Build history of the part. All positions in model axes, mm. A direction names the side the tool comes from. Give positions to 0.01 mm unless a question says otherwise; leave off trailing zeros. Order: outer loops, then holes, each group sorted by start corner. A loop starts at its lowest first (then second) coordinate and runs counter-clockwise, first axis right, second up. Notation, with made-up numbers: (-14, 79.5) - (19, 79.5) arc R31 cw to (19, 117.5) - close; hole circle Ø2 at (48.5, 7). An arc over 180 degrees is marked (long way). One line per item, written item: value.
```python
from build123d import *

# Parameters (mm, degrees)
CUT_EXTRUDE1_DEPTH = 2.54


with BuildPart() as part:
    # Sketch1 → Revolve1 (revolve)
    with BuildSketch(Plane.XY):
        with BuildLine():
            Line((0, 0), (0, 8.7122))
            Line((0, 8.7122), (0.490735938, 8.7122))
            ThreePointArc((0.490735938, 8.7122), (2.913197513, 7.899826069), (4.3561, 5.7912))
            Line((4.3561, 5.7912), (2.4257, 5.7912))
            Line((2.4257, 5.7912), (2.4257, 0))
            Line((2.4257, 0), (0, 0))
        make_face()
    revolve(axis=Axis((0, 0, 0), (0, 1, 0)))

    # Sketch2 → Cut-Extrude1 (cut)
    with BuildSketch(Plane(origin=(0, 8.7122, 0), x_dir=(1, 0, 0), z_dir=(0, 1, 0))):
        Polygon((0, -1.7145), (1.484800555, -0.85725), (1.484800555, 0.85725), (0, 1.7145), (-1.484800555, 0.85725), (-1.484800555, -0.85725), align=None)
    extrude(amount=-CUT_EXTRUDE1_DEPTH, mode=Mode.SUBTRACT)


solid = part.part
```
(1) Pull direction X, two halves, no side cores. Call faces 3 (the face through (-1.485, 7, 0)), 4 (the face through (2.314, 2.855, -0.729)), 5 (the face through (2, 5.791, 2)), 6 (the face through (-0.732, 7.397, -1.292)): +X half, -X half, draft (parallel to the pull), parting line (faces both ways), or undercut.
Completed:
face 3: undercut
face 4: parting line
face 5: draft
face 6: undercut
(2) Slice it at A-A, the plane y = 3.75. Give the cut face in (x, z), and give its area (3 significant figures).
Completed:
outline: circle Ø4.85 at (0, 0)
area: 18.5 mm²
(3) Drill centre lines: line 1 (Y direction, x = 0.5, z = -0.5); line 2 (Z direction, x = 0.5, y = 6.5); line 3 (Z direction, x = 0.75, y = 7.75). Where is each one in solid material? Low to high.
Completed:
line 1: 0 to 6.17
line 2: -4.05 to -1.43, 1.43 to 4.05
line 3: -3.01 to -1.28, 1.28 to 3.01
(4) Pin check, flat tips, straight feed: P1, Ø2.5, axis at x = 0.5, z = 0.5, coming from the +Y side; P2, Ø5, axis at x = -2.5, y = 2.5, coming from the -Z side; P3, Ø1.5, axis at x = -1, y = 7, coming from the -Z side; P4, Ø1.4, axis at y = 8, z = -0.5, coming from the +X side. Stop position of each tip, or through.
Completed:
P1: y = 8.59
P2: z = -2.43
P3: z = -4.11
P4: x = 3.52
(5) 3-axis set-ups, long thin cutter, end or side, ignore diameter. For faces 1 (the face through (0.75, 7.4, -1.28)), 2 (the face through (0, 0, 0)): which of +Z, -Z, +X, -X, +Y, -Y reach the whole face in a straight line?
Completed:
face 1: +Y
face 2: +Z, -Z, +X, -X, -Y
